Geometry check sheet. Reference: the model listing, model coordinates, mm. Face numbers are marked on the shaded views. A direction names the side the tool comes from. Round coordinates to 2 decimals unless told otherwise and drop trailing zeros. Order: outer loops, then holes, each group sorted by start corner. A loop starts at its lowest first (then second) coordinate and runs counter-clockwise, first axis right, second up. Notation, with made-up numbers: M 20,-30 L 49,-30 A14 ccw 49,-11 Z; hole C -16,-23 d7. An arc over 180 degrees is marked long. Answer as a JSON object with one key per item and string values. Group by question number.
```python
from build123d import *

# Parameters (mm, degrees)
SKETCH1_R                    = 5.5
SKETCH1_R_2                  = 6.25
BASE_FLANGE1_DEPTH           = 3
SKETCHED_START               = -3
SKETCHED_BEND1_OUTLINE_R     = 5.5
SKETCHED_BEND1_OUTLINE_R_2   = 6.25
SKETCHED_BEND1_DEPTH         = 3
SKETCHED_START_2             = 0.762
SKETCHED_BEND1_2_OUTLINE_W   = 3
SKETCHED_BEND1_2_OUTLINE_H   = 50
SKETCHED_BEND1_2_DEPTH       = 46.446858709
SKETCHED_START_3             = 47.208858709
SKETCHED_BEND1_3_OUTLINE_R   = 5.5
SKETCHED_BEND1_3_OUTLINE_R_2 = 6.25
SKETCHED_BEND1_3_DEPTH       = 3.762
SKETCHED_BEND1_4_OUTLINE_R   = 5.5
SKETCHED_BEND1_4_OUTLINE_R_2 = 6.25
SKETCHED_BEND1_4_DEPTH       = 0.762
SKETCHED_START_4             = -26
SKETCHED_BEND1_5_DEPTH       = 61
FILLET1_R                    = 18
SKETCH7_R                    = 6.5
CUT_EXTRUDE1_DEPTH           = 10


with BuildPart() as part:
    # Base-Flange1: sheet metal written as solids
    # Sketch1 → Base-Flange1 (new body)
    with BuildSketch(Plane(origin=(0, 0, 0), x_dir=(1, 0, 0), z_dir=(0, 1, 0))):
        with BuildLine():
            Line((45, 25), (-45, 25))
            Line((-45, 25), (-50, 21))
            Line((-50, 21), (-74.5, 21))
            Line((-74.5, 21), (-107.967539406, -17.5))
            ThreePointArc((-107.967539406, -17.5), (-108.177491125, -30.371550102), (-95.532395294, -32.784521956))
            Line((-95.532395294, -32.784521956), (-74.5, -21))
            Line((-74.5, -21), (-50, -21))
            Line((-50, -21), (-45, -25))
            Line((-45, -25), (45, -25))
            Line((45, -25), (50, -21))
            Line((50, -21), (74.5, -21))
            Line((74.5, -21), (95.532395294, -32.784521956))
            ThreePointArc((95.532395294, -32.784521956), (108.177491125, -30.371550102), (107.967539406, -17.5))
            Line((107.967539406, -17.5), (74.5, 21))
            Line((74.5, 21), (50, 21))
            Line((50, 21), (45, 25))
        make_face()
        with Locations(Location((-100.420443604, -24.06059029, 0), (0, 0, 270))):
            Circle(SKETCH1_R, mode=Mode.SUBTRACT)
        with Locations(Location((-74.5, 0, 0), (0, 0, 270))):
            Circle(SKETCH1_R_2, mode=Mode.SUBTRACT)
        with Locations(Location((74.5, 0, 0), (0, 0, 90))):
            Circle(SKETCH1_R_2, mode=Mode.SUBTRACT)
        with Locations(Location((100.420443604, -24.06059029, 0), (0, 0, 90))):
            Circle(SKETCH1_R, mode=Mode.SUBTRACT)
    extrude(amount=-BASE_FLANGE1_DEPTH)

    # Sketched Bend1: read off the stored shape, not the designer's step
    # Sketched Bend1 outline → Sketched Bend1 (cut)
    with BuildSketch(Plane(origin=(0, 0, 0), x_dir=(1, 0, 0), z_dir=(0, 1, 0)).offset(SKETCHED_START)):
        with BuildLine():
            Line((45, 25), (-25, 25))
            Line((-25, 25), (-25, -25))
            Line((-25, -25), (45, -25))
            Line((45, -25), (50, -21))
            Line((50, -21), (74.5, -21))
            Line((74.5, -21), (95.532395294, -32.784521956))
            ThreePointArc((95.532395294, -32.784521956), (108.177491125, -30.371550102), (107.967539406, -17.5))
            Line((107.967539406, -17.5), (74.5, 21))
            Line((74.5, 21), (50, 21))
            Line((50, 21), (45, 25))
        make_face()
        with Locations((100.420443604, -24.06059029)):
            Circle(SKETCHED_BEND1_OUTLINE_R, mode=Mode.SUBTRACT)
        with Locations((74.5, 0)):
            Circle(SKETCHED_BEND1_OUTLINE_R_2, mode=Mode.SUBTRACT)
    extrude(amount=SKETCHED_BEND1_DEPTH, mode=Mode.SUBTRACT)



with BuildPart() as body_2:
    # Sketched Bend1 2 outline → Sketched Bend1 2 (new body)
    with BuildSketch(Plane(origin=(0, 0, 0), x_dir=(1, 0, 0), z_dir=(0, 1, 0)).offset(SKETCHED_START_2)):
        with Locations((-26.5, 0)):
            Rectangle(SKETCHED_BEND1_2_OUTLINE_W, SKETCHED_BEND1_2_OUTLINE_H)
    extrude(amount=SKETCHED_BEND1_2_DEPTH)

    # Sketched Bend1 3 outline → Sketched Bend1 3 (add)
    with BuildSketch(Plane(origin=(0, 0, 0), x_dir=(1, 0, 0), z_dir=(0, 1, 0)).offset(SKETCHED_START_3)):
        with BuildLine():
            Line((-25, -25), (-25, 25))
            Line((-25, 25), (-48.970858709, 25))
            Line((-48.970858709, 25), (-53.970858709, 21))
            Line((-53.970858709, 21), (-78.470858709, 21))
            Line((-78.470858709, 21), (-111.938398115, -17.5))
            ThreePointArc((-111.938398115, -17.5), (-112.148349834, -30.371550102), (-99.503254003, -32.784521956))
            Line((-99.503254003, -32.784521956), (-78.470858709, -21))
            Line((-78.470858709, -21), (-53.970858709, -21))
            Line((-53.970858709, -21), (-48.970858709, -25))
            Line((-48.970858709, -25), (-25, -25))
        make_face()
        with Locations((-104.391302312, -24.06059029)):
            Circle(SKETCHED_BEND1_3_OUTLINE_R, mode=Mode.SUBTRACT)
        with Locations((-78.470858709, 0)):
            Circle(SKETCHED_BEND1_3_OUTLINE_R_2, mode=Mode.SUBTRACT)
    extrude(amount=SKETCHED_BEND1_3_DEPTH)


with BuildPart() as part_1:
    add(part.part)

    add(body_2.part)  # Sketched Bend1 4 merges body 2
    # Sketched Bend1 4 outline → Sketched Bend1 4 (add)
    with BuildSketch(Plane(origin=(0, 0, 0), x_dir=(1, 0, 0), z_dir=(0, 1, 0))):
        with BuildLine():
            Line((-25, -25), (-25, 25))
            Line((-25, 25), (-48.970858709, 25))
            Line((-48.970858709, 25), (-53.970858709, 21))
            Line((-53.970858709, 21), (-78.470858709, 21))
            Line((-78.470858709, 21), (-111.938398115, -17.5))
            ThreePointArc((-111.938398115, -17.5), (-112.148349834, -30.371550102), (-99.503254003, -32.784521956))
            Line((-99.503254003, -32.784521956), (-78.470858709, -21))
            Line((-78.470858709, -21), (-53.970858709, -21))
            Line((-53.970858709, -21), (-48.970858709, -25))
            Line((-48.970858709, -25), (-25, -25))
        make_face()
        with Locations((-104.391302312, -24.06059029)):
            Circle(SKETCHED_BEND1_4_OUTLINE_R, mode=Mode.SUBTRACT)
        with Locations((-78.470858709, 0)):
            Circle(SKETCHED_BEND1_4_OUTLINE_R_2, mode=Mode.SUBTRACT)
    extrude(amount=SKETCHED_BEND1_4_DEPTH)

    # Sketched Bend1 5 outline → Sketched Bend1 5 (cut)
    with BuildSketch(Plane.XY.offset(SKETCHED_START_4)):
        with BuildLine():
            ThreePointArc((-28.762, 50.970858709), (-26.101864289, 49.86899442), (-25, 47.208858709))
            Line((-25, 47.208858709), (-25.000000008, 52))
            Line((-25.000000008, 52), (-116, 52))
            Line((-116, 52), (-116, 50.970858695))
            Line((-116, 50.970858695), (-28.762, 50.970858709))
        make_face()
        with BuildLine():
            ThreePointArc((-25, 0.762), (-26.101864289, -1.898135711), (-28.762, -3))
            Line((-28.762, -3), (-116, -2.999999986))
            Line((-116, -2.999999986), (-116, -4))
            Line((-116, -4), (-25.000000008, -4))
            Line((-25.000000008, -4), (-25, 0.762))
        make_face()
        with BuildLine():
            Line((-28.762, 47.970858709), (-116, 47.970858709))
            Line((-116, 47.970858709), (-116, 47.208858709))
            Line((-116, 47.208858709), (-28, 47.208858709))
            ThreePointArc((-28, 47.208858709), (-28.223184633, 47.747674076), (-28.762, 47.970858709))
        make_face()
        with BuildLine():
            Line((-116, 0), (-28.762, 0))
            ThreePointArc((-28.762, 0), (-28.223184633, 0.223184633), (-28, 0.762))
            Line((-28, 0.762), (-116, 0.762))
            Line((-116, 0.762), (-116, 0))
        make_face()
    extrude(amount=SKETCHED_BEND1_5_DEPTH, mode=Mode.SUBTRACT)

    # Fillet1
    fillet1_edges = [part_1.edges().sort_by_distance(p)[0] for p in [
        (-78.470858709, 49.470858709, 21),
        (-78.470858709, 49.470858709, -21),
        (-74.5, -1.5, -21),
        (-74.5, -1.5, 21),
    ]]
    fillet(fillet1_edges, radius=FILLET1_R)

    # Sketch7 → Cut-Extrude1 (cut)
    with BuildSketch(Plane(origin=(-25, 0, 0), x_dir=(0, 0, -1), z_dir=(1, 0, 0))):
        with Locations(Location((0, 23.985429354, 0), (0, 0, 90))):
            Circle(SKETCH7_R)
    extrude(amount=-CUT_EXTRUDE1_DEPTH, mode=Mode.SUBTRACT)


solid = part_1.part
```
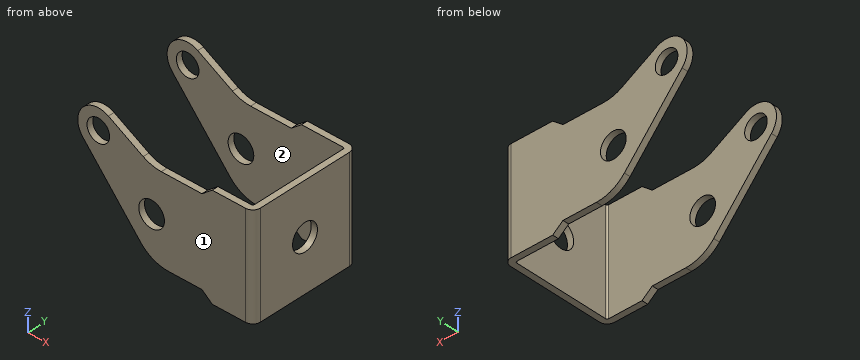
1) Sectioned sample at C-C (z = 0). Record the boundary of the cut face in (x, y).
2) Sectioned sample at D-D (x = -103.5). Record the boundary of the cut face in (y, z).
3) Sectioned sample at A-A (x = -40). Record the boundary of the cut face in (y, z), then the cut area to 3 significant figures.
4) Go/stop test with flat-tipped pins: P1, Ø3.5, axis at x = -64, y = 49, coming from the -Z side; P2, Ø11.5, axis at y = 23.99, z = 0, coming from the +X side; P3, Ø2.5, axis at x = -61.5, y = 50, coming from the +Z side; P4, Ø8, axis at y = 42, z = -11, coming from the -X side. Record where each tip stops, or that it passes through.
5) Set-up check for the marked faces 1 and 2: record each of +Z, -Z, +X, -X, +Y, -Y from which the full face is reachable in a straight line by a thin tool's end or side.
6) Thickness scan on line 1 along Y through (x, z) = (-81, 14.5); line 2 along Y through (x, z) = (-107, 22.5); line 3 along X through (y, z) = (8.5, 3). Record the ranges inside material, lowest first. Write a range as [from, to].
7) Sectioned sample at B-B (y = 25). Record the boundary of the cut face in (x, z).
Final values:
{
 "1": {"outline": "M -96.73,47.97 L -84.72,47.97 L -84.72,50.97 L -96.73,50.97 Z; M -92.76,-3 L -80.75,-3 L -80.75,0 L -92.76,0 Z; M -72.22,47.97 L -28.76,47.97 A0.76 cw -28,47.21 L -28,30.49 L -25,30.49 L -25,47.21 A3.76 ccw -28.76,50.97 L -72.22,50.97 Z; M -68.25,-3 L -28.76,-3 A3.76 ccw -25,0.76 L -25,17.49 L -28,17.49 L -28,0.76 A0.76 cw -28.76,0 L -68.25,0 Z"},
 "2": {"outline": "M -3,12.36 L 0,12.36 L 0,19.5 L -3,19.5 Z; M -3,28.62 L 0,28.62 L 0,33.57 L -3,33.57 Z; M 47.97,7.79 L 50.97,7.79 L 50.97,18.63 L 47.97,18.63 Z; M 47.97,29.49 L 50.97,29.49 L 50.97,34.02 L 47.97,34.02 Z"},
 "3": {"outline": "M -3,-25 L 0,-25 L 0,25 L -3,25 Z; M 47.97,-25 L 50.97,-25 L 50.97,25 L 47.97,25 Z", "area": "300 mm^2"},
 "4": {"P1": "stops at z = -21", "P2": "passes through", "P3": "stops at z = 21", "P4": "stops at x = -28"},
 "5": {"face 1": "+Z, -Z, +X, -X, -Y", "face 2": "+Z, -Z, -X"},
 "6": {"line 1": "y = [-3, 0], [47.97, 50.97]", "line 2": "y = [-3, 0]", "line 3": "x = [-28, -25]"},
 "7": {"outline": "M -28,-25 L -25,-25 L -25,-6.42 L -28,-6.42 Z; M -28,6.42 L -25,6.42 L -25,25 L -28,25 Z"}
}
